Study the drawing (mm; zero at the part's minimum x, y, z) and answer. A direction names the side the tool comes from. Round coordinates to 2 decimals unless told otherwise and drop trailing zeros. Write each loop counter-clockwise with the first axis right and the second up, starting at its lowest first coordinate (ties: lowest second). Pieces come first, ordered by that corner, then holes. Notation, with made-up numbers: (73, 0.5) -> (124, 0.5) arc R24 cw to (124, 26.5) -> close; hole circle Ø6 at (49, 24.25). An arc over 180 degrees is marked (long way). Return JSON: item names as keys, results as strings.
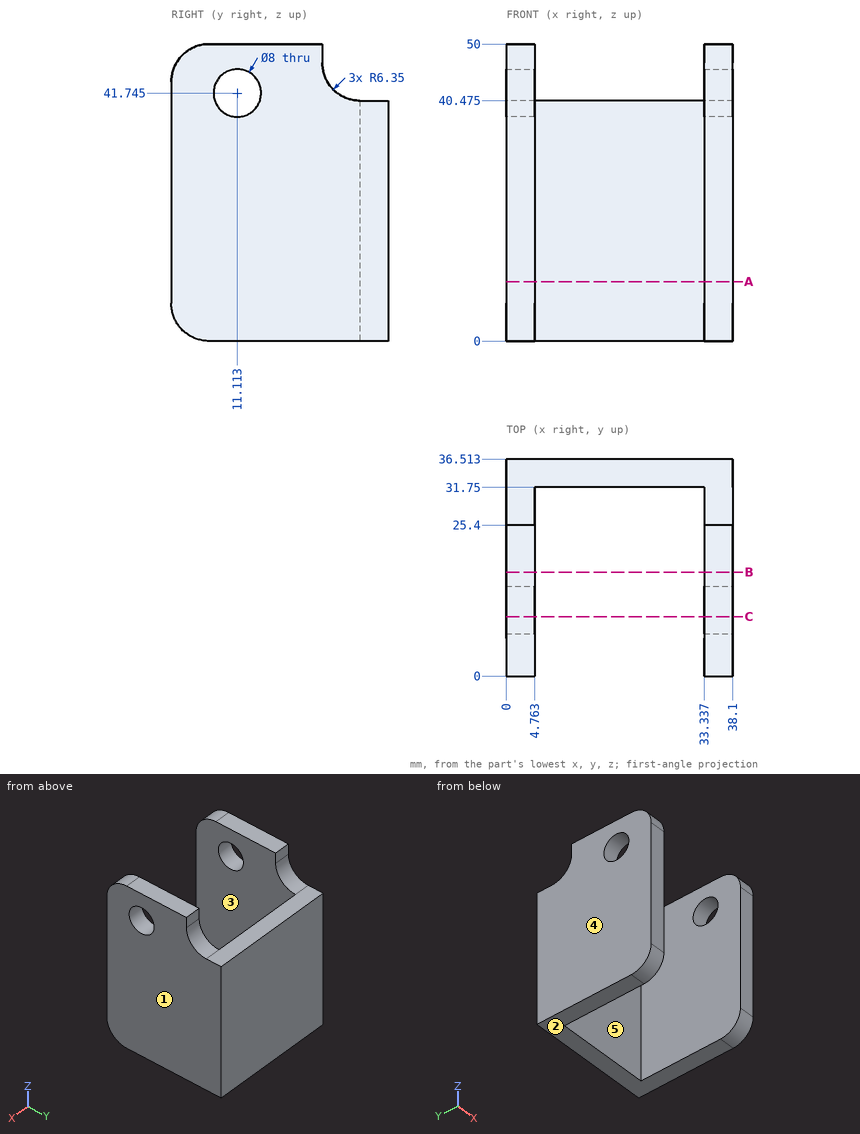
Item 1: For a pull along X with two mould halves and no side action, classify the marked faces 1, 2 and 3 as released by +X, released by -X, zero draft, split by the parting line, or undercut.
Worked answers:
{"face 1": "released by +X", "face 2": "zero draft", "face 3": "undercut"}
Item 2: Section A-A (z = 10) is taken. Give the vertices of the cut face in (x, y), then the cut area to 3 significant figures.
Worked answers:
{"outline": "(0, 0) -> (4.76, 0) -> (4.76, 31.75) -> (33.34, 31.75) -> (33.34, 0) -> (38.1, 0) -> (38.1, 36.51) -> (0, 36.51) -> close", "area": "484 mm2"}
Item 3: Flat-ended cylindrical pins translate along their axes: pin 1 (1 mm diameter, centred on x = 2.5, z = 48.5, fed in from +Y); pin 2 (4 mm diameter, centred on x = 15.5, y = 35.5, fed in from +Z) (1 decimal); pin 3 (1 mm diameter, centred on x = 33.5, z = 30, fed in from -Y). Find the tip coordinate at first contact, or state that the pin passes through.
Worked answers:
{"pin 1": "stops at y = 25.4", "pin 2": "stops at z = 40.5", "pin 3": "stops at y = 0"}
Item 4: Section C-C (y = 10) is taken. Give the vertices of the cut face in (x, z), then the cut area to 3 significant figures.
Worked answers:
{"outline": "(0, 0) -> (4.76, 0) -> (4.76, 37.9) -> (0, 37.9) -> close; (0, 45.59) -> (4.76, 45.59) -> (4.76, 50) -> (0, 50) -> close; (33.34, 0) -> (38.1, 0) -> (38.1, 37.9) -> (33.34, 37.9) -> close; (33.34, 45.59) -> (38.1, 45.59) -> (38.1, 50) -> (33.34, 50) -> close", "area": "403 mm2"}
Item 5: A tool of negligible diameter and unlimited length cuts with its end or side. For the marked faces 4 and 5, from which of +Z, -Z, +X, -X, +Y, -Y can it reach the whole face along a straight path? Write none if from no direction.
Worked answers:
{"face 4": "+Z, -Z, -X, +Y, -Y", "face 5": "+Z, -Z, -Y"}
Item 6: Straight lines are drawn through the part: L1, parallel to X at y = 29, z = 35; L2, parallel to Y at x = 7.5, z = 35; L3, parallel to Y at x = 2.5, z = 43.5 (1 decimal). For each, find the intervals that lie inside material, in ascending order. Write a range as [from, to].
Worked answers:
{"L1": "x = [0, 4.76], [33.34, 38.1]", "L2": "y = [31.75, 36.51]", "L3": "y = [0, 7.5], [14.7, 26.3]"}
Item 7: Section B-B (y = 17.5) is taken. Give the vertices of the cut face in (x, z).
Worked answers:
{"outline": "(0, 0) -> (4.76, 0) -> (4.76, 50) -> (0, 50) -> close; (33.34, 0) -> (38.1, 0) -> (38.1, 50) -> (33.34, 50) -> close"}
